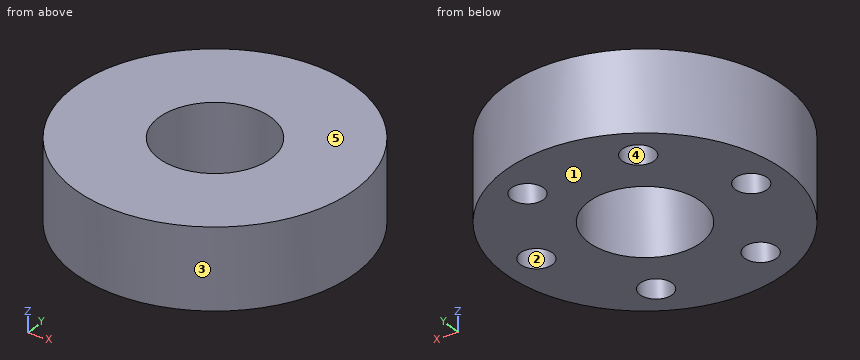
```python
from build123d import *

# Parameters (mm, degrees)
ESQUISSE1_R             = 35
ESQUISSE1_R_2           = 7
BOSS_EXTRU_1_DEPTH      = 20
ESQUISSE2_R             = 14
ENL_V_MAT_EXTRU_1_DEPTH = 5
ESQUISSE3_R             = 4
ENL_V_MAT_EXTRU_3_DEPTH = 5
ESQUISSE8_R             = 14
ENL_V_MAT_EXTRU_4_DEPTH = 25


with BuildPart() as part:
    # Esquisse1 → Boss.-Extru.1 (new body)
    with BuildSketch(Plane.XY):
        Circle(ESQUISSE1_R)
        Circle(ESQUISSE1_R_2, mode=Mode.SUBTRACT)
    extrude(amount=BOSS_EXTRU_1_DEPTH)

    # Esquisse2 → Enlèv. mat.-Extru.1 (cut)
    with BuildSketch(Plane(origin=(0, 0, 0), x_dir=(-1, 0, 0), z_dir=(0, 0, -1))):
        Circle(ESQUISSE2_R)
    extrude(amount=-ENL_V_MAT_EXTRU_1_DEPTH, mode=Mode.SUBTRACT)

    # Esquisse3 → Enlèv. mat.-Extru.3 (cut)
    with BuildSketch(Plane(origin=(0, 0, 0), x_dir=(-1, 0, 0), z_dir=(0, 0, -1))):
        with Locations((-13.588993608, 22.602101614)):
            Circle(ESQUISSE3_R)
        with Locations((13.588993608, 22.602101614)):
            Circle(ESQUISSE3_R)
        with Locations((26.369096609, 0.431843358)):
            Circle(ESQUISSE3_R)
        with Locations((12.841601354, -23.034952123)):
            Circle(ESQUISSE3_R)
        with Locations((-12.82933858, -23.041784138)):
            Circle(ESQUISSE3_R)
        with Locations((-26.369096609, 0.431843358)):
            Circle(ESQUISSE3_R)
    extrude(amount=-ENL_V_MAT_EXTRU_3_DEPTH, mode=Mode.SUBTRACT)

    # Esquisse8 → Enlèv. mat.-Extru.4 (cut)
    with BuildSketch(Plane(origin=(0, 0, 0), x_dir=(-1, 0, 0), z_dir=(0, 0, -1))):
        Circle(ESQUISSE8_R)
    extrude(amount=-ENL_V_MAT_EXTRU_4_DEPTH, mode=Mode.SUBTRACT)


solid = part.part
```
Source: CAD feature listing. Evaluate the final solid. Frame: model axes, mm. Face numbers are marked on the shaded views. A direction names the side the tool comes from. Round coordinates to 2 decimals unless told otherwise and drop trailing zeros. Loops run counter-clockwise (first coordinate to the right, second up) from the corner with the lowest first, then second, coordinate; pieces in that order, holes last. Notation, with made-up numbers: M 34.5,-4 L 57.5,-4 A33 cw 57.5,33 Z; hole C 13.25,-13.5 d7. An arc over 180 degrees is marked long. Use a Markdown table: item, result. Add a question column.
1. Cut plane A-A, the plane x = 0. Output: boundary loops of the cut face in (y, z), and give its area (3 significant figures).
2. Contact query for flat-ended pins moving along their axis: pin 1 (2.5 mm diameter, centred on x = -12.5, y = 22.5, fed in from -Z); pin 2 (22.5 mm diameter, centred on x = 0, y = 0, fed in from +Z); pin 3 (6.5 mm diameter, centred on x = -13.5, y = -22.5, fed in from -Z); pin 4 (2 mm diameter, centred on x = -27, z = 14.5, fed in from -Y). Output: stop coordinate, or through.
3. Pull-direction query (X, two-part tool) for the marked faces 3, 4 and 5; classes: +X half, -X half, draft (parallel to the pull), parting line (faces both ways), or undercut.
4. Cut plane B-B, the plane y = -10. Output: boundary loops of the cut face in (x, z), and give its area (3 significant figures).
5. Cut plane D-D, the plane x = -12.5. Output: boundary loops of the cut face in (y, z).
6. Ray query, line 1 along X through (y, z) = (-19.5, 2); line 2 along Z through (x, y) = (-15, -25); line 3 along X through (y, z) = (-8, 1). Return the intervals inside material, ascending. Write a range as [from, to].
7. Cut plane C-C, the plane z = 17. Output: boundary loops of the cut face in (x, y).
8. Set-up query: the marked faces 1 and 2. Return all of +Z, -Z, +X, -X, +Y, -Y with unobstructed straight access to the full face (end or side cutting, diameter ignored); none if empty.
Solution:
| question | item | result |
|---|---|---|
| 1 | outline | M -35,0 L -14,0 L -14,20 L -35,20 Z; M 14,0 L 35,0 L 35,20 L 14,20 Z |
| 1 | area | 840 mm2 |
| 2 | pin 1 | stops at z = 5 |
| 2 | pin 2 | passes through |
| 2 | pin 3 | stops at z = 0 |
| 2 | pin 4 | stops at y = -23.43 |
| 3 | face 3 | parting line |
| 3 | face 4 | undercut |
| 3 | face 5 | draft |
| 4 | outline | M -33.54,0 L -9.8,0 L -9.8,20 L -33.54,20 Z; M 9.8,0 L 33.54,0 L 33.54,20 L 9.8,20 Z |
| 4 | area | 950 mm2 |
| 5 | outline | M -32.69,0 L -27.02,0 L -27.02,5 L -19.05,5 L -19.05,0 L -6.3,0 L -6.3,20 L -32.69,20 Z; M 6.3,0 L 18.75,0 L 18.75,5 L 26.45,5 L 26.45,0 L 32.69,0 L 32.69,20 L 6.3,20 Z |
| 6 | line 1 | x = [-29.06, -14.71], [-10.97, 10.97], [14.69, 29.06] |
| 6 | line 2 | z = [5, 20] |
| 6 | line 3 | x = [-34.07, -11.49], [11.49, 34.07] |
| 7 | outline | C 0,0 d70; hole C 0,0 d28 |
| 8 | face 1 | -Z, +X, -X, +Y, -Y |
| 8 | face 2 | -Z |
